```python
from build123d import *

# Parameters (mm, degrees)
SKETCH1_R          = 11.1
EXTRUDE1_DEPTH     = 12.7
SKETCH3_R          = 1.85
CUT_EXTRUDE1_DEPTH = 13.7
SKETCH6_R          = 3.95
EXTRUDE3_DEPTH     = 2.5
SKETCH7_R          = 3.95
EXTRUDE4_DEPTH     = 2.5
SKETCH8_R          = 2.45
CUT_EXTRUDE2_DEPTH = 18.7


with BuildPart() as part:
    # Sketch1 → Extrude1 (new body)
    with BuildSketch(Plane.XY):
        Circle(SKETCH1_R)
    extrude(amount=-EXTRUDE1_DEPTH)

    # Sketch3 → Cut-Extrude1 (cut, through all)
    with BuildSketch(Plane.XY):
        with Locations((8, 0)):
            Circle(SKETCH3_R)
        with Locations((-8, 0)):
            Circle(SKETCH3_R)
        with Locations((0, -8)):
            Circle(SKETCH3_R)
        with Locations((0, 8)):
            Circle(SKETCH3_R)
    extrude(amount=-CUT_EXTRUDE1_DEPTH, mode=Mode.SUBTRACT)

    # Sketch6 → Extrude3 (add)
    with BuildSketch(Plane.XY):
        Circle(SKETCH6_R)
    extrude(amount=EXTRUDE3_DEPTH)

    # Sketch7 → Extrude4 (add)
    with BuildSketch(Plane(origin=(0, 0, -12.7), x_dir=(-1, 0, 0), z_dir=(0, 0, -1))):
        Circle(SKETCH7_R)
    extrude(amount=EXTRUDE4_DEPTH)

    # Sketch8 → Cut-Extrude2 (cut, through all)
    with BuildSketch(Plane.XY.offset(2.5)):
        Circle(SKETCH8_R)
    extrude(amount=-CUT_EXTRUDE2_DEPTH, mode=Mode.SUBTRACT)


solid = part.part
```
Work out the finished part from the listing and answer in its coordinate system (mm). A direction names the side the tool comes from. Round coordinates to 2 decimals unless told otherwise and drop trailing zeros. Write each loop counter-clockwise with the first axis right and the second up, starting at its lowest first coordinate (ties: lowest second). Pieces come first, ordered by that corner, then holes. Notation, with made-up numbers: (-39, 51.25) - (16, 51.25) arc R27 cw to (16, 85.25) - close; hole circle Ø3 at (46, 34.25). An arc over 180 degrees is marked (long way). Return JSON: item names as keys, results as strings. Group by question number.
Q1. Each of these flat-tipped pins is pushed along its axis until it touches: pin 1 Ø1 at (x, z) = (1, -2.5) entering from +Y; pin 2 Ø3 at (y, z) = (5, -10) entering from +X; pin 3 Ø2 at (x, z) = (-8, -0.5) entering from -Y. Where does it stop, or does it pass through?
Q2. The part is cut by section C-C on x = -8. Write down the section's boundary in (y, z).
Q3. The mould has two halves that part along Y. Classify faces 1 (the flat face through (-2, 2, -15.2)), 2 (the cylindrical face through (5.97, 9.36, -6.26)), 3 (the cylindrical face through (0.854, -9.641, -6.261)), 4 (the cylindrical face through (-0.401, 6.194, -6.261)): released by +Y, released by -Y, zero draft, split by the parting line, or undercut.
Q4. For faces 5 (the flat face through (5, 0, 0)), 6 (the cylindrical face through (-9.468, -1.126, -6.261)), 7 (the flat face through (5, 0, -12.7)), determine the directions among +Z, -Z, +X, -X, +Y, -Y from which every point of the face is accessible in a straight line to the end or side of a thin tool.
Q5. Find the intervals of material crossed by L1, parallel to Y at x = 0, z = -3.5; L2, parallel to X at y = 1, z = -0.75; L3, parallel to Y at x = -6.5, z = -12, in increasing order.
Q6. The part is cut by section A-A on y = 0. Write down the section's boundary in (x, z).
Solved:
{
 "1": {"pin 1": "y = 11.09", "pin 2": "x = 10.53", "pin 3": "y = -8.61"},
 "2": {"outline": "(-7.69, -12.7) - (-1.85, -12.7) - (-1.85, 0) - (-7.69, 0) - close; (1.85, -12.7) - (7.69, -12.7) - (7.69, 0) - (1.85, 0) - close"},
 "3": {"face 1": "zero draft", "face 2": "split by the parting line", "face 3": "undercut", "face 4": "undercut"},
 "4": {"face 5": "+Z", "face 6": "+Z, -Z", "face 7": "-Z"},
 "5": {"L1": "-11.1 to -9.85, -6.15 to -2.45, 2.45 to 6.15, 9.85 to 11.1", "L2": "-11.05 to -9.56, -6.44 to -2.24, 2.24 to 6.44, 9.56 to 11.05", "L3": "-9 to -1.08, 1.08 to 9"},
 "6": {"outline": "(-11.1, -12.7) - (-9.85, -12.7) - (-9.85, 0) - (-11.1, 0) - close; (-6.15, -12.7) - (-3.95, -12.7) - (-3.95, -15.2) - (-2.45, -15.2) - (-2.45, 2.5) - (-3.95, 2.5) - (-3.95, 0) - (-6.15, 0) - close; (2.45, -15.2) - (3.95, -15.2) - (3.95, -12.7) - (6.15, -12.7) - (6.15, 0) - (3.95, 0) - (3.95, 2.5) - (2.45, 2.5) - close; (9.85, -12.7) - (11.1, -12.7) - (11.1, 0) - (9.85, 0) - close"}
}
